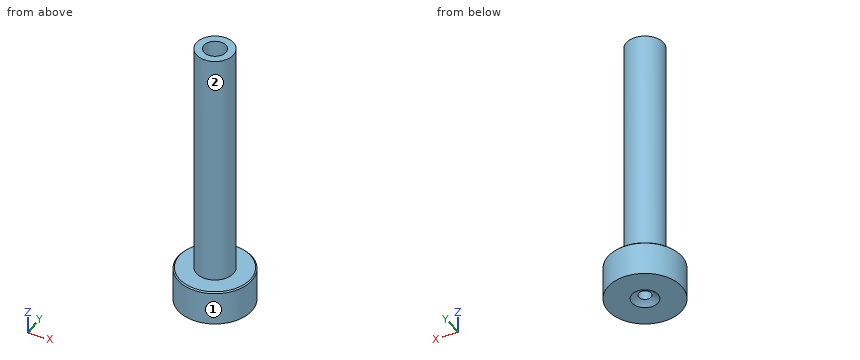
from build123d import *

# Parameters (mm, degrees)
F0_R     = 23.749
F1_DEPTH = 22.225
F2_R     = 11.9634
F3_DEPTH = 176.784
F4_R     = 3.9755383952
F5_DEPTH = 176.785
F5_TAPER = -1
F8_SIZE  = 0.7874


with BuildPart() as f1:
    # F0 (on Top) → F1 (new body)
    with BuildSketch(Plane.XY):
        Circle(F0_R)
    extrude(amount=F1_DEPTH)

    # F2 (on Top) → F3 (join)
    with BuildSketch(Plane.XY):
        Circle(F2_R)
    extrude(amount=F3_DEPTH)

    # F4 (on Top) → F5 (cut, through all)
    with BuildSketch(Plane.XY):
        Circle(F4_R)
    extrude(amount=F5_DEPTH, taper=F5_TAPER, mode=Mode.SUBTRACT)

    # F6 (on Front) → F7 (revolve, cut)
    with BuildSketch(Plane.XZ):
        with BuildLine():
            Line((0, -9.525), (0, 0))
            Line((0, 0), (0, 3.175))
            ThreePointArc((0, 3.175), (-12.7, -9.525), (0, -22.225))
            Line((0, -22.225), (0, -9.525))
        make_face()
    revolve(axis=Axis((0, 0, -4.7625), (0, 0, -1)), mode=Mode.SUBTRACT)

    # F8
    f8_edges = [f1.edges().sort_by_distance(p)[0] for p in [
        (-23.749, 0, 22.225),
    ]]
    chamfer(f8_edges, length=F8_SIZE)


solid = f1.part
Work out the finished part from the listing and answer in its coordinate system (mm). Face numbers are marked on the shaded views. A direction names the side the tool comes from. Round coordinates to 2 decimals unless told otherwise and drop trailing zeros. Write each loop counter-clockwise with the first axis right and the second up, starting at its lowest first coordinate (ties: lowest second). Pieces come first, ordered by that corner, then holes. Notation, with made-up numbers: M -31.5,-31 L 7.5,-31 A24 ccw 7.5,-9 Z; hole C 58.5,23 d6. An arc over 180 degrees is marked long. Use a Markdown table: item, result.
1) Which of the six approach directions +Z, -Z, +X, -X, +Y, -Y give full straight-line access (tool end or side, diameter ignored) to the marked faces 1 and 2?
Taken from the geometry:
| item | result |
|---|---|
| face 1 | +Z, -Z |
| face 2 | +Z |
2) The part is cut by section A-A on z = 119. Give the vertices of the cut face in (x, y), plus the area to 3 significant figures.
Taken from the geometry:
| item | result |
|---|---|
| outline | C 0,0 d23.93; hole C 0,0 d12.11 |
| area | 335 mm2 |
3) Flat-ended cylindrical pins translate along their axes: pin 1 (3 mm diameter, centred on x = 4, z = 27.5, fed in from +Y); pin 2 (2 mm diameter, centred on x = 7, z = 108.5, fed in from +Y); pin 3 (6 mm diameter, centred on x = -7.5, z = 150.5, fed in from +Y). Find the tip coordinate at first contact, or state that the pin passes through.
Taken from the geometry:
| item | result |
|---|---|
| pin 1 | stops at y = 11.7 |
| pin 2 | stops at y = 10.35 |
| pin 3 | stops at y = 11.08 |
4) Consider line 1 (Z direction, x = -11, y = -17) (3 decimals); line 2 (X direction, y = -3, z = 67); line 3 (Y direction, x = 3, z = 90). Determine where each line is inside the solid, lowest interval first. Write a range as [from, to].
Taken from the geometry:
| item | result |
|---|---|
| line 1 | z = [0, 22.225] |
| line 2 | x = [-11.58, -4.18], [4.18, 11.58] |
| line 3 | y = [-11.58, -4.67], [4.67, 11.58] |
5) The part is cut by section B-B on z = 48. Give the vertices of the cut face in (x, y).
Taken from the geometry:
| item | result |
|---|---|
| outline | C 0,0 d23.93; hole C 0,0 d9.63 |
